```python
from build123d import *

# Parameters (mm, degrees)
F1_DEPTH = 2
F3_DEPTH = 2.001
F4_R     = 2
F6_DEPTH = 2.001


with BuildPart() as f1:
    # F0 (on Front) → F1 (new body)
    with BuildSketch(Plane.XZ):
        with BuildLine():
            Line((80, 5), (0, 5))
            ThreePointArc((0, 5), (-5, 0), (0, -5))
            Line((0, -5), (80, -5))
            Line((80, -5), (80, 5))
        make_face()
        with BuildLine():
            Line((66, -2.1), (0, -2.1))
            ThreePointArc((0, -2.1), (-2.1, 0), (0, 2.1))
            Line((0, 2.1), (66, 2.1))
            ThreePointArc((66, 2.1), (68.1, 0), (66, -2.1))
        make_face(mode=Mode.SUBTRACT)
    extrude(amount=F1_DEPTH)

    # F2 (on face) → F3 (cut, through all)
    with BuildSketch(Plane.XZ.offset(2)):
        Polygon((73, 5), (71, 5), (72, 4), align=None)
        Polygon((73, -5), (72, -4), (71, -5), align=None)
    extrude(amount=-F3_DEPTH, mode=Mode.SUBTRACT)

    # F4
    f4_edges = [f1.edges().sort_by_distance(p)[0] for p in [
        (80, -1, 5),
        (80, -1, -5),
    ]]
    fillet(f4_edges, radius=F4_R)

    # F5 (on face) → F6 (cut, through all)
    with BuildSketch(Plane.XZ.offset(2)):
        with BuildLine():
            Line((80, -0.1), (80, 0.1))
            Line((80, 0.1), (68.0976176963, 0.1))
            ThreePointArc((68.0976176963, 0.1), (68.1, 0), (68.0976176963, -0.1))
            Line((68.0976176963, -0.1), (80, -0.1))
        make_face()
    extrude(amount=-F6_DEPTH, mode=Mode.SUBTRACT)


solid = f1.part
```
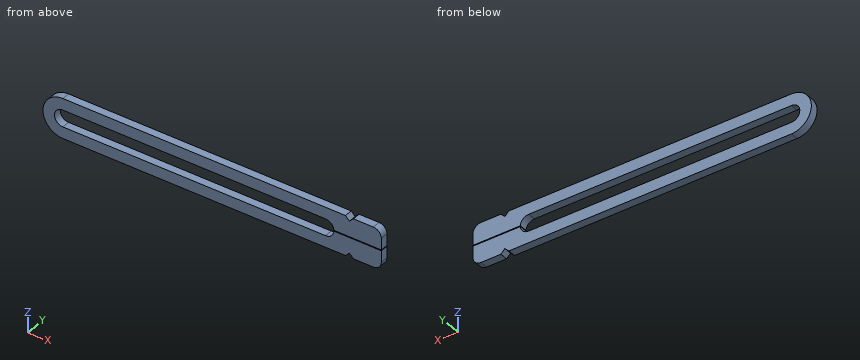
Design review of the part built by this model. Coordinates are the model's own, in mm. Round coordinates to 2 decimals unless told otherwise and drop trailing zeros. Write each loop counter-clockwise with the first axis right and the second up, starting at its lowest first coordinate (ties: lowest second). Pieces come first, ordered by that corner, then holes. Notation, with made-up numbers: (60.25, 13.25) -> (100.25, 13.25) arc R10 ccw to (100.25, 26.25) -> close; hole circle Ø5 at (44, -17.5). An arc over 180 degrees is marked (long way). Write item = value, one per line. Start each with the question number.
1) Take a section at B-B, the plane y = -1.4. State the section outline as (x, z) points, plus the area to 3 significant figures.
2) Clearance check with flat-ended pins moving along their axes: pin 1 (5 mm diameter, centred on x = 29.5, z = -0.5, fed in from +Y); pin 2 (0.6 mm diameter, centred on x = 72.5, y = -1.5, fed in from -Z). State where each tip first meets the part, or that it passes through.
3) Wall thickness on probe 1 along Z at (x, y) = (31.5, -1.1); probe 2 along X at (y, z) = (-0.35, 0.25); probe 3 along Z at (x, y) = (72, -0.75): over which ranges is each line inside the solid? List them lowest first. Write a range as from..to.
4) Take a section at C-C, the plane z = -1. State the section outline as (x, y) points, plus the area to 3 significant figures.
5) Take a section at A-A, the plane x = 14. State the section outline as (y, z) points.
Results list:
q1.outline = (0, -5) -> (71, -5) -> (72, -4) -> (73, -5) -> (78, -5) arc R2 ccw to (80, -3) -> (80, -0.1) -> (68.1, -0.1) arc R2.1 cw to (66, -2.1) -> (0, -2.1) arc R2.1 cw to (0, 2.1) -> (66, 2.1) arc R2.1 cw to (68.1, 0.1) -> (80, 0.1) -> (80, 3) arc R2 ccw to (78, 5) -> (73, 5) -> (72, 4) -> (71, 5) -> (0, 5) arc R5 ccw to start
q1.area = 542 mm²
q2.pin_1 = 0
q2.pin_2 = -4.8
q3.probe_1 = -5..-2.1, 2.1..5
q3.probe_2 = -4.99..-2.09, 68.09..80
q3.probe_3 = -4..-0.1, 0.1..4
q4.outline = (-4.9, -2) -> (-1.85, -2) -> (-1.85, 0) -> (-4.9, 0) -> close; (67.85, -2) -> (80, -2) -> (80, 0) -> (67.85, 0) -> close
q4.area = 30.4 mm²
q5.outline = (-2, -5) -> (0, -5) -> (0, -2.1) -> (-2, -2.1) -> close; (-2, 2.1) -> (0, 2.1) -> (0, 5) -> (-2, 5) -> close
